Geometry: see drawing. Coordinates: mm, zero at the bounding-box minimum. Give positions to 0.01 mm unless a question says otherwise; leave off trailing zeros. Write each loop counter-clockwise with the first axis right and the second up, starting at its lowest first coordinate (ties: lowest second). Pieces come first, ordered by that corner, then holes. Notation, with made-up numbers: (-22, 67.5) - (34, 67.5) arc R18 ccw to (34, 86.5) - close; hole circle Ø8 at (52.25, 79). An arc over 180 degrees is marked (long way). Use CSV: the item, a comma, the result in double quotes. Start each with the question number.
(1) Line query: probe 1 along X at (y, z) = (1.3, 8.25) (1 decimal); probe 2 along Z at (x, y) = (5, 0.35) (1 decimal); probe 3 along X at (y, z) = (0.1, 6) (1 decimal). Output: solid intervals per line, ascending. Write a range as [from, to].
(2) First-contact query: pin 1 Ø5 at (x, z) = (80.4, 7.75) entering from +Y. Flat tip, straight axial feed; report the tip coordinate or a pass-through.
(3) Section B-B on y = 1.2. Output: boundary loops of the cut face in (x, z) (1 decimal), and give its area (3 significant figures).
(4) Section A-A on x = 12.7. Output: boundary loops of the cut face in (y, z) (1 decimal).
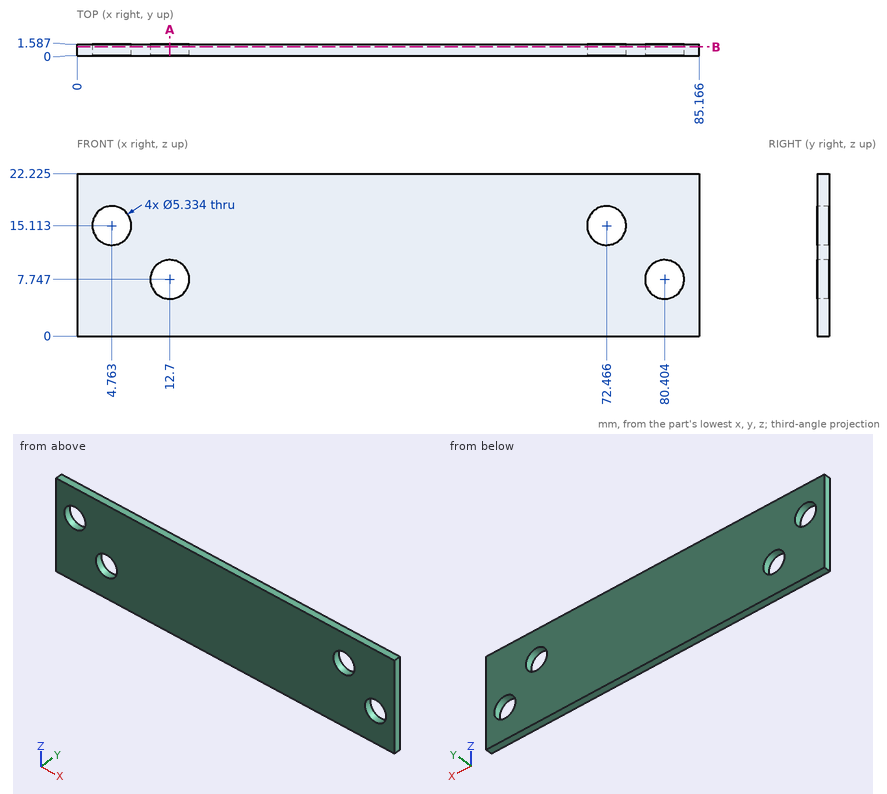
Check values:
1,probe 1,"x = [0, 10.1], [15.3, 77.8], [83, 85.2]"
1,probe 2,"z = [0, 12.5], [17.8, 22.2]"
1,probe 3,"x = [0, 10.7], [14.7, 78.4], [82.4, 85.2]"
2,pin 1,"passes through"
3,outline,"(0, 0) - (85.2, 0) - (85.2, 22.2) - (0, 22.2) - close; hole circle Ø5.3 at (4.8, 15.1); hole circle Ø5.3 at (12.7, 7.7); hole circle Ø5.3 at (72.5, 15.1); hole circle Ø5.3 at (80.4, 7.7)"
3,area,"1,800 mm²"
4,outline,"(0, 0) - (1.6, 0) - (1.6, 5.1) - (0, 5.1) - close; (0, 10.4) - (1.6, 10.4) - (1.6, 22.2) - (0, 22.2) - close"
